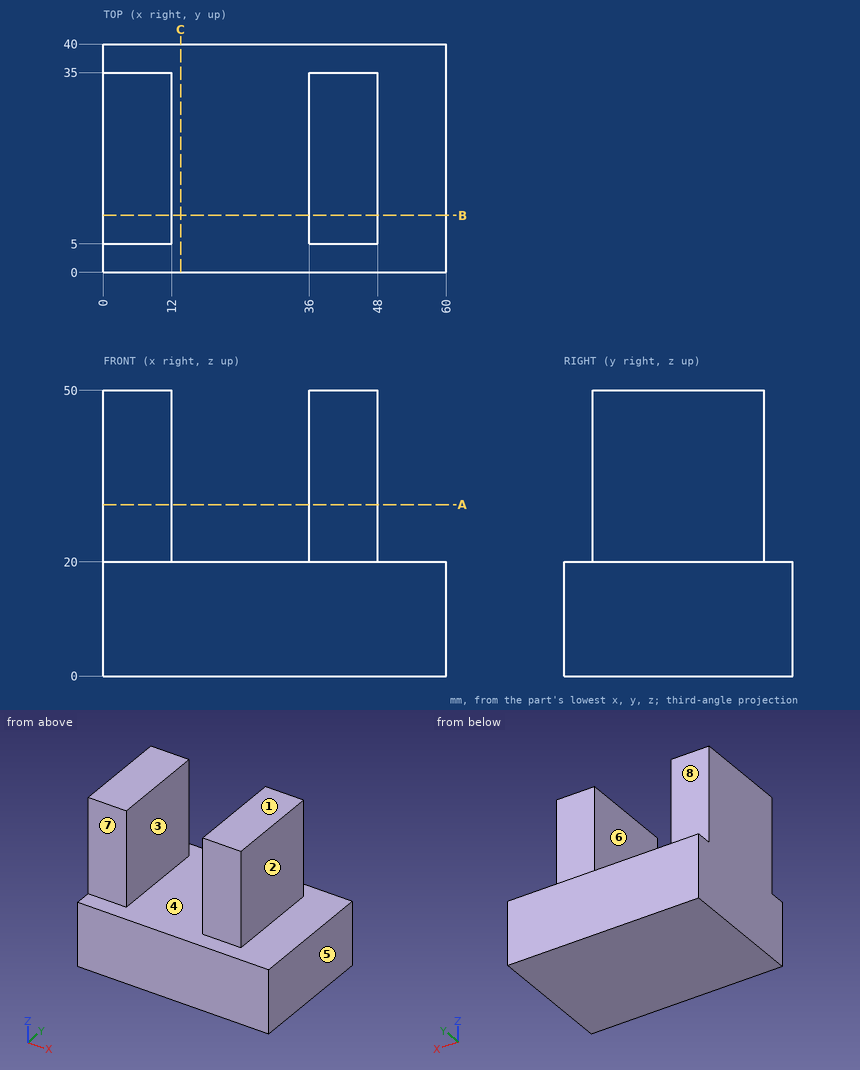
Verification items for this drawing (mm, ordinates from the low corner). A direction names the side the tool comes from. Give positions to 0.01 mm unless a question says otherwise; leave off trailing zeros. Loops run counter-clockwise (first coordinate to the right, second up) from the corner with the lowest first, then second, coordinate; pieces in that order, holes last.
1. Release check for a two-part mould opening along X. For the marked faces 1, 2, 3 and 4 record: +X half, -X half, draft (parallel to the pull), parting line (faces both ways), or undercut.
Derived:
face 1: draft
face 2: +X half
face 3: undercut
face 4: undercut
2. Cross-section at A-A on z = 30. Record the cut outline in (x, y).
Derived:
outline: (0, 5) - (12, 5) - (12, 35) - (0, 35) - close; (36, 5) - (48, 5) - (48, 35) - (36, 35) - close
3. Material ranges on probe 1 along X at (y, z) = (28.5, 37); probe 2 along Z at (x, y) = (39.5, 36); probe 3 along Y at (x, z) = (47, 32), recorded low to high.
Derived:
probe 1: x = 0 to 12, 36 to 48
probe 2: z = 0 to 20
probe 3: y = 5 to 35
4. Cross-section at B-B on y = 10. Record the cut outline in (x, z), and give its area (3 significant figures).
Derived:
outline: (0, 0) - (60, 0) - (60, 20) - (48, 20) - (48, 50) - (36, 50) - (36, 20) - (12, 20) - (12, 50) - (0, 50) - close
area: 1,920 mm2
5. Tool access check on the marked faces 5, 6, 7 and 8. Record the directions out of +Z, -Z, +X, -X, +Y, -Y that give a thin tool (end or side, any length) a straight path to the whole face; none if there is none.
Derived:
face 5: +Z, -Z, +X, +Y, -Y
face 6: +Z, +Y, -Y
face 7: +Z, +X, -X, -Y
face 8: +Z, +X, -X, +Y
6. Go/stop test with flat-tipped pins: P1, Ø4, axis at y = 25, z = 35.5, coming from the +X side; P2, Ø6, axis at x = 42.5, z = 42.5, coming from the -Y side; P3, Ø6, axis at x = 42.5, z = 33.5, coming from the +Y side. Record where each tip stops, or that it passes through.
Derived:
P1: stops at x = 48
P2: stops at y = 5
P3: stops at y = 35
7. Cross-section at C-C on x = 13.5. Record the cut outline in (y, z).
Derived:
outline: (0, 0) - (40, 0) - (40, 20) - (0, 20) - close
